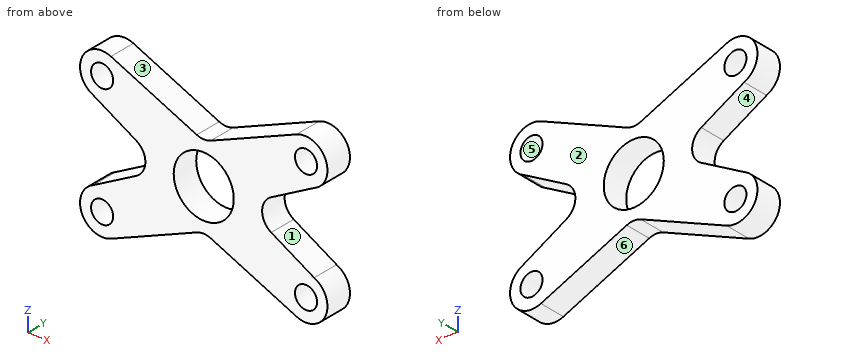
Autodesk Inventor part; units mm, degrees
ref_plane "YZ Plane" through (0, 0, 0) normal (1, 0, 0) x (0, 1, 0)
ref_plane "XZ Plane" through (0, 0, 0) normal (0, 1, 0) x (-1, 0, 0)
ref_plane "XY Plane" through (0, 0, 0) normal (0, 0, 1) x (1, 0, 0)
sketch "Boceto1" plane through (0, 0, 0) normal (0, 1, 0) x (-1, 0, 0)
  arc A0 (22.0076, -15.7946) -> (23.9924, -11.2054) centre (23, -13.5) ccw
  arc A1 (23.9924, -2.2946) -> (22.0076, 2.2946) centre (23, 0) ccw
  arc A2 (0.9924, 2.2946) -> (-0.9924, -2.2946) centre (0, 0) ccw
  arc A3 (-0.9924, -11.2054) -> (0.9924, -15.7946) centre (0, -13.5) ccw
  line L0 (12.2939, -1.9066) -> (22.0076, 2.2946)
  line L1 (19.1337, -5.0031) -> (23.9924, -2.2946)
  line L2 (19.1337, -8.4969) -> (23.9924, -11.2054)
  line L3 (0.9924, 2.2946) -> (10.7061, -1.9066)
  line L4 (-0.9924, -2.2946) -> (3.8663, -5.0031)
  line L5 (3.8663, -8.4969) -> (-0.9924, -11.2054)
  line L6 (12.2939, -11.5934) -> (22.0076, -15.7946)
  line L7 (10.7061, -11.5934) -> (0.9924, -15.7946)
  circle A4 centre (11.5, -6.75) radius 3.4
  arc A5 (19.1337, -5.0031) -> (19.1337, -8.4969) centre (20.1075, -6.75) ccw
  arc A6 (10.7061, -1.9066) -> (12.2939, -1.9066) centre (11.5, -0.071) ccw
  arc A7 (3.8663, -8.4969) -> (3.8663, -5.0031) centre (2.8925, -6.75) ccw
  arc A8 (12.2939, -11.5934) -> (10.7061, -11.5934) centre (11.5, -13.429) ccw
  circle A9 centre (23, 0) radius 1.25
  circle A10 centre (23, -13.5) radius 1.25
  circle A11 centre (-0.0735, 0) radius 1.25
  circle A12 centre (-0.0735, -13.5) radius 1.25
extrude "Extrusión1" add sketch "Boceto1" along normal blind 3
properties part number "Extension2"
Verification items for the finished model (mm, model axes). Face numbers are marked on the shaded views. A direction names the side the tool comes from. Coordinates: 2 decimals unless noted, no trailing zeros. Order: outer loops, then holes, each group sorted by start corner. A loop starts at its lowest first (then second) coordinate and runs counter-clockwise, first axis right, second up. Notation, with made-up numbers: M -29.5,40.5 L -2.5,40.5 A15 ccw -2.5,66.5 Z; hole C -31.5,13 d6. An arc over 180 degrees is marked long. One line per item, written item: value. Start each with the question number.
Item 1: Sectioned sample at D-D on x = -23. Record the cut outline in (y, z).
Item 2: Sectioned sample at B-B on x = -3.5. Record the cut outline in (y, z).
Item 3: Depth check by flat-ended pin: P1, Ø1.5, axis at x = -5.5, y = 2, coming from the -Z side; P2, Ø1, axis at y = 2.5, z = -9.5, coming from the +X side; P3, Ø2, axis at x = -12, z = -8, coming from the -Y side; P4, Ø1.5, axis at y = 2.5, z = -9, coming from the -X side. Enter the tip coordinate at first touch or a pass-through.
Item 4: Access from +Z, -Z, +X, -X, +Y, -Y to the whole of each face (thin tool, end or side, straight path). Record for the marked faces 4, 5 and 6.
Item 5: Mould release check, pull along X, two halves, no side actions. Record for the marked faces 1, 2 and 3: pulls with the +X half, pulls with the -X half, needs draft (parallel to the pull), parting line crosses it, or undercut.
Item 6: Thickness scan on probe 1 along Z at (x, y) = (0.5, 2.6); probe 2 along Z at (x, y) = (-22, 2.05); probe 3 along Z at (x, y) = (-9.5, 1.65). Record the ranges inside material, lowest first.
Item 7: Sectioned sample at A-A on z = -6.75. Record the cut outline in (x, y).
Calculated:
1. outline: M 0,-16 L 3,-16 L 3,-14.75 L 0,-14.75 Z; M 0,-12.25 L 3,-12.25 L 3,-10.65 L 0,-10.65 Z; M 0,-2.85 L 3,-2.85 L 3,-1.25 L 0,-1.25 Z; M 0,1.25 L 3,1.25 L 3,2.5 L 0,2.5 Z
2. outline: M 0,-14.71 L 3,-14.71 L 3,-8.7 L 0,-8.7 Z; M 0,-4.8 L 3,-4.8 L 3,1.21 L 0,1.21 Z
3. P1: z = -14.17
3. P2: x = -1.17
3. P3: through
3. P4: x = -21.38
4. face 4: -X, +Y, -Y
4. face 5: +Y, -Y
4. face 6: -Z, +Y, -Y
5. face 1: pulls with the +X half
5. face 2: needs draft
5. face 3: undercut
6. probe 1: -15.95 to -14.67, -12.33 to -10.93, -2.57 to -1.17, 1.17 to 2.45
6. probe 2: -15.79 to -14.25, -12.75 to -10.09, -3.41 to -0.75, 0.75 to 2.29
6. probe 3: -12.12 to -9.5, -4 to -1.38
7. outline: M -18.11,0 L -14.9,0 L -14.9,3 L -18.11,3 Z; M -8.1,0 L -4.89,0 L -4.89,3 L -8.1,3 Z
